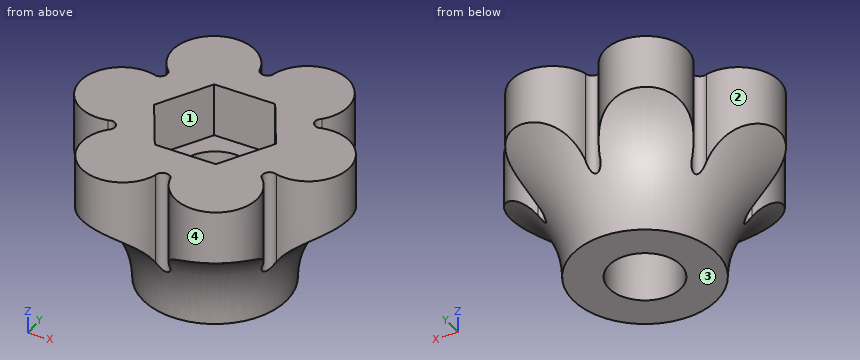
```python
from build123d import *

# Parameters (mm, degrees)
SKETCH008_R     = 3.35
PAD004_DEPTH    = 15
POCKET002_DEPTH = 5


with BuildPart() as part:
    # Sketch008 → Pad004 (new body)
    with BuildSketch(Plane.XY):
        with BuildLine():
            ThreePointArc((7.1470904861, 4.890715447), (6.25, 10.8253175473), (0.6619385767, 8.6349196476))
            ThreePointArc((-0.6619385767, 8.6349196476), (0, 7.9978308267), (0.6619385767, 8.6349196476))
            ThreePointArc((-0.6619385767, 8.6349196476), (-6.25, 10.8253175473), (-7.1470904861, 4.890715447))
            ThreePointArc((-7.8090290628, 3.7442042006), (-6.9263246711, 3.9989154133), (-7.1470904861, 4.890715447))
            ThreePointArc((-7.8090290628, 3.7442042006), (-12.5, 0), (-7.8090290628, -3.7442042006))
            ThreePointArc((-7.1470904861, -4.890715447), (-6.9263246711, -3.9989154133), (-7.8090290628, -3.7442042006))
            ThreePointArc((-7.1470904861, -4.890715447), (-6.25, -10.8253175473), (-0.6619385767, -8.6349196476))
            ThreePointArc((0.6619385767, -8.6349196476), (0, -7.9978308267), (-0.6619385767, -8.6349196476))
            ThreePointArc((0.6619385767, -8.6349196476), (6.25, -10.8253175473), (7.1470904861, -4.890715447))
            ThreePointArc((7.8090290628, -3.7442042006), (6.9263246711, -3.9989154133), (7.1470904861, -4.890715447))
            ThreePointArc((7.8090290628, -3.7442042006), (12.5, 0), (7.8090290628, 3.7442042006))
            ThreePointArc((7.1470904861, 4.890715447), (6.9263246711, 3.9989154133), (7.8090290628, 3.7442042006))
        make_face()
        Circle(SKETCH008_R, mode=Mode.SUBTRACT)
    extrude(amount=PAD004_DEPTH)

    # Sketch009 (on Face15 of Pad004) → Pocket002 (cut)
    with BuildSketch(Plane.XY.offset(15)):
        Polygon((2.825, -4.8930435314), (5.65, 0), (2.825, 4.8930435314), (-2.825, 4.8930435314), (-5.65, 0), (-2.825, -4.8930435314), align=None)
    extrude(amount=-POCKET002_DEPTH, mode=Mode.SUBTRACT)

    # Sketch010 → Groove (revolve, cut)
    with BuildSketch(Plane.XZ):
        with BuildLine():
            ThreePointArc((12.5, 10), (8.2549337817, 5.7801384066), (6.7, 0))
            Line((6.7, 0), (13.5, 0))
            Line((13.5, 0), (13.5, 10))
            Line((13.5, 10), (12.5, 10))
        make_face()
    revolve(axis=Axis((0, 0, 0), (0, 0, 1)), mode=Mode.SUBTRACT)


solid = part.part
```
The listing builds one solid part. Answer for the finished solid, in the listing's coordinates (mm). Face numbers are marked on the shaded views. A direction names the side the tool comes from. Give positions to 0.01 mm unless a question says otherwise; leave off trailing zeros. Order: outer loops, then holes, each group sorted by start corner. A loop starts at its lowest first (then second) coordinate and runs counter-clockwise, first axis right, second up. Notation, with made-up numbers: (-14.5, 12.5) -> (40.5, 12.5) arc R21 ccw to (40.5, 51.5) -> close; hole circle Ø3 at (41, 84.5). An arc over 180 degrees is marked (long way). Answer as CSV lines item,"result". Start each with the question number.
Q1. A cutting plane is placed at B-B (z = 8). Determine the outline of the cut face in (x, y), then the cut area to 3 significant figures.
Q2. Determine the mould class of the marked faces 3 and 4 for opening direction Y: pulls with the +Y half, pulls with the -Y half, needs draft (parallel to the pull), parting line crosses it, or undercut.
Q3. A cutting plane is placed at D-D (z = 3.5). Determine the outline of the cut face in (x, y).
Q4. Which of the six approach directions +Z, -Z, +X, -X, +Y, -Y give full straight-line access (tool end or side, diameter ignored) to the marked faces 1 and 2?
Q5. A cutting plane is placed at C-C (x = 7.5). Count the separate pieces of the cut face and the enclosed holes in it, then the cut area to 3 significant figures.
Q6. Find the intervals of material crossed by L1, parallel to Y at x = 0, z = 5.75; L2, parallel to X at y = 0, z = 4.25; L3, parallel to Y at x = 0, z = 2.75, in increasing order.
Q7. Given pin 1 (4 mm diameter, centred on x = -0.5, z = 12.5, fed in from +Y); pin 2 (4 mm diameter, centred on x = 4, z = 6.5, fed in from +Y); pin 3 (2.5 mm diameter, centred on x = 1.5, z = 12.5, fed in from -Y), each flat-ended and moving along its own axis, determine where each tip first touches the part or whether it passes through.
Q8. A cutting plane is placed at A-A (x = 0). Determine the outline of the cut face in (y, z).
Results found:
1,outline,"(-9.17, -3.81) arc R3.84 ccw to (-7.81, -3.74) arc R0.66 cw to (-7.15, -4.89) arc R3.84 ccw to (-7.88, -6.04) arc R9.93 ccw to (-1.29, -9.85) arc R3.84 ccw to (-0.66, -8.63) arc R0.66 cw to (0.66, -8.63) arc R3.84 ccw to (1.29, -9.85) arc R9.93 ccw to (7.88, -6.04) arc R3.84 ccw to (7.15, -4.89) arc R0.66 cw to (7.81, -3.74) arc R3.84 ccw to (9.17, -3.81) arc R9.93 ccw to (9.17, 3.81) arc R3.84 ccw to (7.81, 3.74) arc R0.66 cw to (7.15, 4.89) arc R3.84 ccw to (7.88, 6.04) arc R9.93 ccw to (1.29, 9.85) arc R3.84 ccw to (0.66, 8.63) arc R0.66 cw to (-0.66, 8.63) arc R3.84 ccw to (-1.29, 9.85) arc R9.93 ccw to (-7.88, 6.04) arc R3.84 ccw to (-7.15, 4.89) arc R0.66 cw to (-7.81, 3.74) arc R3.84 ccw to (-9.17, 3.81) arc R9.93 ccw to start; hole circle Ø6.7 at (0, 0)"
1,area,"256 mm2"
2,face 3,"needs draft"
2,face 4,"undercut"
3,outline,"circle Ø14.49 at (0, 0); hole circle Ø6.7 at (0, 0)"
4,face 1,"+Z"
4,face 2,"+Z, -Z"
5,separate pieces,"3"
5,enclosed holes,"0"
5,area,"130 mm2"
6,L1,"-8 to -3.35, 3.35 to 8"
6,L2,"-7.51 to -3.35, 3.35 to 7.51"
6,L3,"-7.03 to -3.35, 3.35 to 7.03"
7,pin 1,"y = 10.88"
7,pin 2,"y = 9.77"
7,pin 3,"y = -11"
8,outline,"(-8, 5.31) arc R11.52 cw to (-6.7, 0) -> (-3.35, 0) -> (-3.35, 10) -> (-4.89, 10) -> (-4.89, 15) -> (-8, 15) -> close; (3.35, 0) -> (6.7, 0) arc R11.52 cw to (8, 5.31) -> (8, 15) -> (4.89, 15) -> (4.89, 10) -> (3.35, 10) -> close"
